Geometry: final body of the model. Coordinates: model frame, mm. Face numbers are marked on the shaded views. Coordinates: 2 decimals unless noted, no trailing zeros. Loops run counter-clockwise (first coordinate to the right, second up) from the corner with the lowest first, then second, coordinate; pieces in that order, holes last. Notation, with made-up numbers: (38, -12.75) - (46, -12.75) arc R27 cw to (46, 14.25) - close; hole circle Ø1 at (83.5, 70.25). An arc over 180 degrees is marked (long way). Answer in a Markdown table with one row per item.
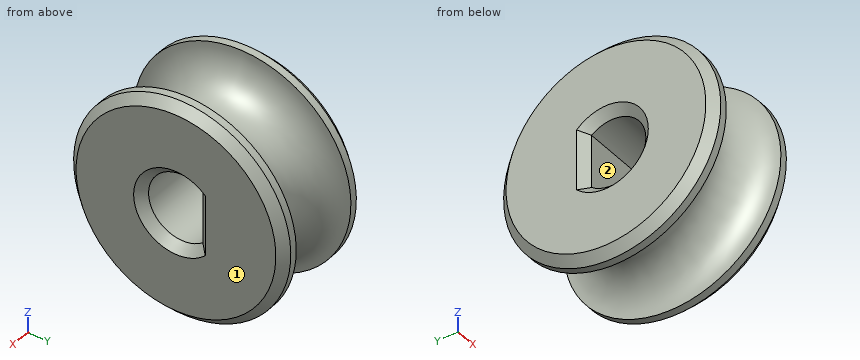
from build123d import *

# Parameters (mm, degrees)
CUT_EXTRUDE1_DEPTH = 11.307764064
CHAMFER1_SIZE      = 0.4


with BuildPart() as part:
    # Sketch1 → Revolve1 (revolve)
    with BuildSketch(Plane.XY, mode=Mode.PRIVATE) as revolve1_sk:
        with BuildLine():
            Line((1.75, 2.5), (2.5, 2.5))
            Line((2.5, 2.5), (2.5, -2.5))
            Line((2.5, -2.5), (-2.5, -2.5))
            Line((-2.5, -2.5), (-2.5, 2.5))
            Line((-2.5, 2.5), (-1.75, 2.5))
            ThreePointArc((-1.75, 2.5), (0, 0.75), (1.75, 2.5))
        make_face()
    revolve(revolve1_sk.sketch.rotate(Axis((-2.5, -2.5, 0), (1, 0, 0)), 90), axis=Axis((-2.5, -2.5, 0), (1, 0, 0)))

    # Sketch2 → Cut-Extrude1 (cut, through all)
    with BuildSketch(Plane(origin=(2.5, 0, 0), x_dir=(0, 0, -1), z_dir=(1, 0, 0))):
        with BuildLine():
            Line((-1.224744871, -1.55), (1.224744871, -1.55))
            ThreePointArc((1.224744871, -1.55), (0, -4.05), (-1.224744871, -1.55))
        make_face()
    extrude(amount=-CUT_EXTRUDE1_DEPTH, mode=Mode.SUBTRACT)

    # Chamfer1
    chamfer1_edges = [part.edges().sort_by_distance(p)[0] for p in [
        (-2.5, -4.05, 0),
        (-2.5, -1.55, 0),
        (2.5, -4.05, 0),
        (2.5, -1.55, 0),
        (-2.5, -2.5, -5),
        (2.5, -2.5, -5),
    ]]
    chamfer(chamfer1_edges, length=CHAMFER1_SIZE)


solid = part.part
(1) Cut plane A-A on z = 0. Output: boundary loops of the cut face in (x, y), then the cut area to 3 significant figures.
Verdict:
| item | result |
|---|---|
| outline | (-2.5, -7.1) - (-2.1, -7.5) - (-1.75, -7.5) arc R1.75 cw to (1.75, -7.5) - (2.1, -7.5) - (2.5, -7.1) - (2.5, -4.45) - (2.1, -4.05) - (-2.1, -4.05) - (-2.5, -4.45) - close; (-2.5, -1.15) - (-2.1, -1.55) - (2.1, -1.55) - (2.5, -1.15) - (2.5, 2.1) - (2.1, 2.5) - (1.75, 2.5) arc R1.75 cw to (-1.75, 2.5) - (-2.1, 2.5) - (-2.5, 2.1) - close |
| area | 27.2 mm² |
(2) First-contact query: pin 1 Ø3 at (x, z) = (0, -3.5) entering from -Y; pin 2 Ø0.7 at (x, z) = (1, 0.5) entering from -Y; pin 3 Ø1.5 at (x, z) = (-1.5, 3.5) entering from +Y. Flat tips, straight axial feed; report the tip coordinate or a pass-through.
Verdict:
| item | result |
|---|---|
| pin 1 | stops at y = -5.17 |
| pin 2 | stops at y = -6.36 |
| pin 3 | stops at y = 1.65 |
(3) Pull-direction query (Z, two-part tool) for the marked faces 1 and 2; classes: pulls with the +Z half, pulls with the -Z half, needs draft (parallel to the pull), parting line crosses it, or undercut.
Verdict:
| item | result |
|---|---|
| face 1 | needs draft |
| face 2 | undercut |
(4) Cut plane C-C on x = 0.1. Output: boundary loops of the cut face in (y, z).
Verdict:
| item | result |
|---|---|
| outline | circle Ø6.51 at (-2.5, 0); hole (-1.55, -1.22) - (-1.55, 1.22) arc R1.55 ccw (long way) to start |
(5) Cut plane B-B on x = -1.35. Output: boundary loops of the cut face in (y, z).
Verdict:
| item | result |
|---|---|
| outline | circle Ø7.77 at (-2.5, 0); hole (-1.55, -1.22) - (-1.55, 1.22) arc R1.55 ccw (long way) to start |
(6) Ray query, probe 1 along Z at (x, y) = (-0.65, 0.5); probe 2 along Z at (x, y) = (-0.05, -1.75); probe 3 along X at (y, z) = (-1.5, -3.5). Return the intervals inside material, ascending.
Verdict:
| item | result |
|---|---|
| probe 1 | z = -1.55 to 1.55 |
| probe 2 | z = -3.16 to -1.36, 1.36 to 3.16 |
| probe 3 | x = -2.5 to -1.1, 1.1 to 2.5 |
